Build history of the part. All positions in model axes, mm. A direction names the side the tool comes from. Coordinates: 2 decimals unless noted, no trailing zeros. Write each loop counter-clockwise with the first axis right and the second up, starting at its lowest first coordinate (ties: lowest second). Pieces come first, ordered by that corner, then holes.
```python
from build123d import *

# Parameters (mm, degrees)
EXTRUDE_1_DEPTH     = 16
SKETCH_2_R          = 10
SKETCH_2_R_2        = 7.5
CUT_EXTRUDE_1_DEPTH = 16
SKETCH_3_W          = 8
SKETCH_3_H          = 40
CUT_EXTRUDE_2_DEPTH = 65


with BuildPart() as part:
    # 草图1 → 凸台-拉伸1 (new body)
    with BuildSketch(Plane(origin=(0, 0, 0), x_dir=(0, 0, -1), z_dir=(1, 0, 0))):
        with BuildLine():
            ThreePointArc((20, 0), (0, 20), (-20, 0))
            Line((-20, 0), (-15, -180))
            ThreePointArc((-15, -180), (0, -195), (15, -180))
            Line((15, -180), (20, 0))
        make_face()
    extrude(amount=EXTRUDE_1_DEPTH)

    # 草图2 → 切除-拉伸1 (cut)
    with BuildSketch(Plane(origin=(16, 0, 0), x_dir=(0, 0, -1), z_dir=(1, 0, 0))):
        Circle(SKETCH_2_R)
        with Locations((0, -180)):
            Circle(SKETCH_2_R_2)
    extrude(amount=-CUT_EXTRUDE_1_DEPTH, mode=Mode.SUBTRACT)

    # 草图3 → 切除-拉伸2 (cut)
    with BuildSketch(Plane(origin=(0, -230, 0), x_dir=(1, 0, 0), z_dir=(0, 1, 0))):
        with Locations((7.927431522, 0)):
            Rectangle(SKETCH_3_W, SKETCH_3_H)
    extrude(amount=CUT_EXTRUDE_2_DEPTH, mode=Mode.SUBTRACT)


solid = part.part
```
1. Probe line 1 along Y through (x, z) = (2.05, 0); line 2 along Y through (x, z) = (11.5, 0); line 3 along Y through (x, z) = (3.25, 4). List the from-to ranges inside material, lowest first.
Computed values:
line 1: y = -195 to -187.5, -172.5 to -10, 10 to 20
line 2: y = -165 to -10, 10 to 20
line 3: y = -194.46 to -186.34, -173.66 to -9.17, 9.17 to 19.6
2. Saw through at A-A on z = 0. List the corners of the cut face in (x, y), plus the area to 3 significant figures.
Computed values:
outline: (0, -195) - (3.93, -195) - (3.93, -187.5) - (0, -187.5) - close; (0, -172.5) - (3.93, -172.5) - (3.93, -165) - (11.93, -165) - (11.93, -172.5) - (16, -172.5) - (16, -10) - (0, -10) - close; (0, 10) - (16, 10) - (16, 20) - (0, 20) - close; (11.93, -195) - (16, -195) - (16, -187.5) - (11.93, -187.5) - close
area: 2,760 mm2
3. Saw through at C-C on z = -12. List the corners of the cut face in (x, y).
Computed values:
outline: (0, -189) - (3.93, -189) - (3.93, -165) - (11.93, -165) - (11.93, -189) - (16, -189) - (16, 16) - (0, 16) - close
4. 3-axis set-ups, long thin cutter, end or side, ignore diameter. For faces 5 (the face through (11.927, -176.9, 7.1)), 6 (the face through (2, -195, 0)): which of +Z, -Z, +X, -X, +Y, -Y reach the whole face in a straight line?
Computed values:
face 5: +Z, -Z, -Y
face 6: +X, -X, -Y
5. Flat gauge pins, fed straight in: pin 1 (9 mm diameter, centred on y = -180, z = 0, fed in from +X); pin 2 (4 mm diameter, centred on x = 8, z = -6, fed in from -Y); pin 3 (6 mm diameter, centred on x = 11, y = -3.5, fed in from -Z); pin 4 (6 mm diameter, centred on x = 12, y = -45.5, fed in from +Z). Where does each tip first touch, or does it go through?
Computed values:
pin 1: passes through
pin 2: stops at y = -165
pin 3: stops at z = -19.99
pin 4: stops at z = 18.82
6. Saw through at D-D on y = -69. List the corners of the cut face in (x, z), plus the area to 3 significant figures.
Computed values:
outline: (0, -18.08) - (16, -18.08) - (16, 18.08) - (0, 18.08) - close
area: 579 mm2
7. Saw through at B-B on x = 14. List the corners of the cut face in (y, z).
Computed values:
outline: (-180, -15) - (0, -20) arc R20 ccw to (0, 20) - (-180, 15) arc R15 ccw to start; hole circle Ø15 at (-180, 0); hole circle Ø20 at (0, 0)
8. Mould opens along Y. For faces 1 (the face through (8, 20, 0)), 2 (the face through (3.927, -176.9, 7.1)), 3 (the face through (14, -195, 0)), 4 (the face through (8.11, -9.76, 2.17)) say: +Y half, -Y half, draft (parallel to the pull), parting line (faces both ways), or undercut.
Computed values:
face 1: +Y half
face 2: draft
face 3: -Y half
face 4: undercut
